Geometry check sheet. Reference: the model listing, model coordinates, mm. Face numbers are marked on the shaded views. A direction names the side the tool comes from. Coordinates: 2 decimals unless noted, no trailing zeros. Loops run counter-clockwise (first coordinate to the right, second up) from the corner with the lowest first, then second, coordinate; pieces in that order, holes last.
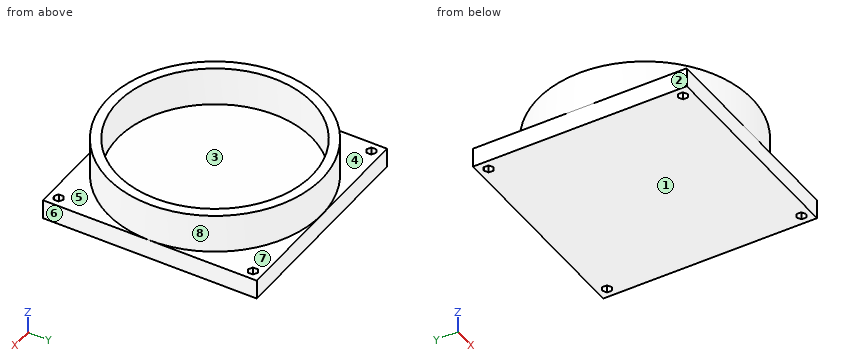
from build123d import *

# Parameters (mm, degrees)
SKETCH2_R           = 55
BOSS_EXTRUDE2_DEPTH = 30
SKETCH5_R           = 50
CUT_EXTRUDE2_DEPTH  = 21
SKETCH6_W           = 110
SKETCH6_H           = 110
BOSS_EXTRUDE3_DEPTH = 10
CUT_EXTRUDE5_DEPTH  = 23


with BuildPart() as part:
    # Sketch2 → Boss-Extrude2 (new body)
    with BuildSketch(Plane.XY):
        Circle(SKETCH2_R)
    extrude(amount=BOSS_EXTRUDE2_DEPTH)

    # Sketch5 → Cut-Extrude2 (cut)
    with BuildSketch(Plane.XY.offset(30)):
        Circle(SKETCH5_R)
    extrude(amount=-CUT_EXTRUDE2_DEPTH, mode=Mode.SUBTRACT)

    # Sketch6 → Boss-Extrude3 (add)
    with BuildSketch(Plane.XY):
        Rectangle(SKETCH6_W, SKETCH6_H)
    extrude(amount=BOSS_EXTRUDE3_DEPTH)

    # Sketch7 → Cut-Extrude5 (cut)
    with BuildSketch(Plane.XY):
        Polygon((-47.826827432, 48.764151713), (-47.843137704, 51.264098507), (-50.016310272, 52.499946794), (-52.173172568, 51.235848287), (-52.156862296, 48.735901493), (-49.983689728, 47.500053206), align=None)
        Polygon((50.080599261, 47.501299586), (52.204237665, 48.8204508), (52.123638405, 51.319151214), (49.919400739, 52.498700414), (47.795762335, 51.1795492), (47.876361595, 48.680848786), align=None)
        Polygon((52.165063509, -51.25), (52.165063509, -48.75), (50, -47.5), (47.834936491, -48.75), (47.834936491, -51.25), (50, -52.5), align=None)
        Polygon((-49.98483432, -52.499954), (-47.827393488, -51.236843136), (-47.842559168, -48.736889136), (-50.01516568, -47.500046), (-52.172606512, -48.763156864), (-52.157440832, -51.263110864), align=None)
    extrude(amount=CUT_EXTRUDE5_DEPTH, mode=Mode.SUBTRACT)


solid = part.part
(1) Sectioned sample at C-C on z = 23.5. Record the cut outline in (x, y), and give its area (3 significant figures).
Findings:
outline: circle Ø110 at (0, 0); hole circle Ø100 at (0, 0)
area: 1,650 mm2
(2) Scan lines: L1, parallel to Y at x = 0, z = 24; L2, parallel to Z at x = 30.5, y = -25; L3, parallel to X at y = 6, z = 27.5. Record each from-to range of solid material in increasing order.
Findings:
L1: y = -55 to -50, 50 to 55
L2: z = 0 to 10
L3: x = -54.67 to -49.64, 49.64 to 54.67
(3) Sectioned sample at A-A on x = -6. Record the cut outline in (y, z).
Findings:
outline: (-55, 0) - (55, 0) - (55, 10) - (54.67, 10) - (54.67, 30) - (49.64, 30) - (49.64, 10) - (-49.64, 10) - (-49.64, 30) - (-54.67, 30) - (-54.67, 10) - (-55, 10) - close
(4) Draft check along X on the marked faces 1, 2 and 3. Enter one of: +X half, -X half, draft (parallel to the pull), parting line (faces both ways), or undercut.
Findings:
face 1: draft
face 2: -X half
face 3: undercut
(5) Sectioned sample at B-B on y = 41. Record the cut outline in (x, z), and give its area (3 significant figures).
Findings:
outline: (-55, 0) - (55, 0) - (55, 10) - (36.66, 10) - (36.66, 30) - (28.62, 30) - (28.62, 10) - (-28.62, 10) - (-28.62, 30) - (-36.66, 30) - (-36.66, 10) - (-55, 10) - close
area: 1,420 mm2
(6) Access from +Z, -Z, +X, -X, +Y, -Y to the whole of each face (thin tool, end or side, straight path). Record for the marked faces 4, 5, 6, 7 and 8.
Findings:
face 4: +Z, -X, +Y
face 5: +Z, +X, -Y
face 6: +Z, -Z, +X, +Y, -Y
face 7: +Z, +X, +Y
face 8: +Z
(7) Gauge pin test, flat ends, axial feed: pin 1 Ø5 at (x, z) = (26.5, 23.5) entering from -Y; pin 2 Ø10 at (x, y) = (29, -34.5) entering from +Z; pin 3 Ø1.5 at (x, y) = (-20.5, -32.5) entering from +Z; pin 4 Ø5 at (x, z) = (-9.5, 18) entering from -Y. Record the tip position at first contact, or that the pin passes through.
Findings:
pin 1: stops at y = -49.49
pin 2: stops at z = 30
pin 3: stops at z = 10
pin 4: stops at y = -54.55
